Design review of the part built by this model. Coordinates are the model's own, in mm. Face numbers are marked on the shaded views. A direction names the side the tool comes from. Coordinates: 2 decimals unless noted, no trailing zeros. Order: outer loops, then holes, each group sorted by start corner. A loop starts at its lowest first (then second) coordinate and runs counter-clockwise, first axis right, second up. Notation, with made-up numbers: (-27.75, 7.25) -> (18.25, 7.25) arc R32 cw to (18.25, 34.25) -> close; hole circle Ø3 at (16.25, -3). An arc over 180 degrees is marked (long way). Write item = value, one per line.
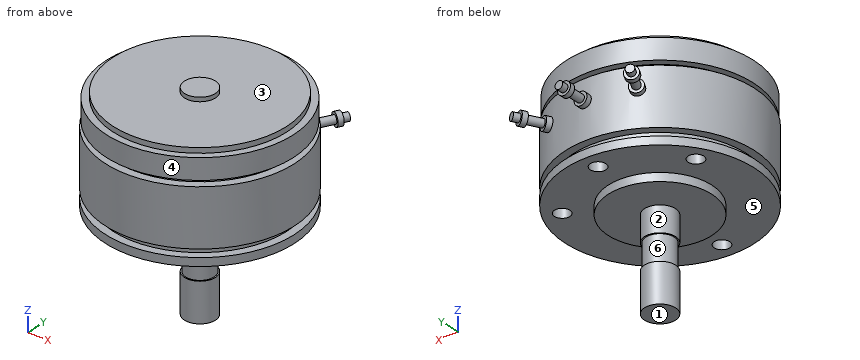
```python
from build123d import *

# Parameters (mm, degrees)
SKETCH_5_R                 = 3
SKETCH_5_R_2               = 2.75
EXTRUDE_3_DEPTH            = 19
SKETCH_5_3_R               = 10
SKETCH_5_3_R_2             = 3
EXTRUDE_4_DEPTH            = 1.6
CUT_EXTRUDE_START          = 6.5
SKETCH_5_4_R               = 3
SKETCH_5_4_R_2             = 2.75
CUT_EXTRUDE_5_DEPTH        = 5
SKETCH_6_R                 = 0.75
EXTRUDE_5_DEPTH            = 24.5
EXTRUDE_START              = 18.207141
SKETCH_6_4_R               = 1.25
SKETCH_6_4_R_2             = 0.75
EXTRUDE_10_DEPTH           = 5.042859
SKETCH_6_5_R               = 1.25
SKETCH_6_5_R_2             = 0.75
CUT_EXTRUDE_6_DEPTH        = 22.25
SKETCH_6_6_R               = 1.25
SKETCH_6_6_R_2             = 0.75
EXTRUDE_11_DEPTH           = 19.25
PATTERN_CIRCULAR_1_ANGLE   = 28
PATTERN_CIRCULAR_1_2_ANGLE = 28
SKETCH_7_R                 = 1.5
CUT_EXTRUDE_7_DEPTH        = 3
EXTRUDE_START_2            = 0.8
SKETCH_8_R                 = 3
EXTRUDE_12_DEPTH           = 0.8


with BuildPart() as part:
    # Sketch 4 → Revolve 1 (revolve)
    with BuildSketch(Plane(origin=(0, 0, 0), x_dir=(0, 0, -1), z_dir=(1, 0, 0)), mode=Mode.PRIVATE) as revolve_1_sk:
        Polygon((0, 0), (0, 16.75), (1, 16.75), (1, 18.05), (5, 18.05), (5, 16.75), (6, 16.75), (6, 18.25), (16.93, 18.25), (16.93, 16.75), (18.43, 16.75), (18.43, 18.25), (20, 18.25), (20, 0), align=None)
    revolve(revolve_1_sk.sketch.rotate(Axis((0, 0, 42.478286457), (0, 0, -1)), 90), axis=Axis((0, 0, 42.478286457), (0, 0, -1)))

    # Sketch 5 → Extrude 3 (add)
    # profile 1 of 2: a face of its own
    with BuildSketch(Plane(origin=(0, 0, -20), x_dir=(-1, 0, 0), z_dir=(0, 0, -1))):
        Circle(SKETCH_5_R)
        Circle(SKETCH_5_R_2, mode=Mode.SUBTRACT)
    # profile 2 of 2: a face of its own
    with BuildSketch(Plane(origin=(0, 0, -20), x_dir=(-1, 0, 0), z_dir=(0, 0, -1))):
        Circle(SKETCH_5_R_2)
    extrude(amount=EXTRUDE_3_DEPTH)

    # Sketch 5_3 → Extrude 4 (add)
    with BuildSketch(Plane(origin=(0, 0, -20), x_dir=(-1, 0, 0), z_dir=(0, 0, -1))):
        Circle(SKETCH_5_3_R)
        Circle(SKETCH_5_3_R_2, mode=Mode.SUBTRACT)
    extrude(amount=EXTRUDE_4_DEPTH)

    # Sketch 5_4 → Cut-Extrude 5 (cut)
    with BuildSketch(Plane(origin=(0, 0, -20), x_dir=(-1, 0, 0), z_dir=(0, 0, -1)).offset(CUT_EXTRUDE_START)):
        Circle(SKETCH_5_4_R)
        Circle(SKETCH_5_4_R_2, mode=Mode.SUBTRACT)
    extrude(amount=CUT_EXTRUDE_5_DEPTH, mode=Mode.SUBTRACT)

    # Sketch 6 → Extrude 5 (add)
    with BuildSketch(Plane(origin=(0, 0, 0), x_dir=(1, 0, 0), z_dir=(0, 1, 0))):
        with Locations(Location((0, 10, 0), (0, 0, 90))):
            Circle(SKETCH_6_R)
    extrude(amount=EXTRUDE_5_DEPTH)

    # Sketch 6_4 → Extrude 10 (add)
    with BuildSketch(Plane(origin=(0, 0, 0), x_dir=(1, 0, 0), z_dir=(0, 1, 0)).offset(EXTRUDE_START)):
        with Locations(Location((0, 10, 0), (0, 0, 90))):
            Circle(SKETCH_6_4_R)
        with Locations(Location((0, 10, 0), (0, 0, 270))):
            Circle(SKETCH_6_4_R_2, mode=Mode.SUBTRACT)
    extrude(amount=EXTRUDE_10_DEPTH)

    # Sketch 6_5 → Cut-Extrude 6 (cut)
    with BuildSketch(Plane(origin=(0, 0, 0), x_dir=(1, 0, 0), z_dir=(0, 1, 0))):
        with Locations(Location((0, 10, 0), (0, 0, 90))):
            Circle(SKETCH_6_5_R)
        with Locations(Location((0, 10, 0), (0, 0, 270))):
            Circle(SKETCH_6_5_R_2, mode=Mode.SUBTRACT)
    extrude(amount=CUT_EXTRUDE_6_DEPTH, mode=Mode.SUBTRACT)

    # Sketch 6_6 → Extrude 11 (add)
    with BuildSketch(Plane(origin=(0, 0, 0), x_dir=(1, 0, 0), z_dir=(0, 1, 0))):
        with Locations(Location((0, 10, 0), (0, 0, 90))):
            Circle(SKETCH_6_6_R)
        with Locations(Location((0, 10, 0), (0, 0, 270))):
            Circle(SKETCH_6_6_R_2, mode=Mode.SUBTRACT)
    extrude(amount=EXTRUDE_11_DEPTH)


with BuildPart() as body_2:
    # Pattern Circular 1: read off the stored shape, not the designer's step
    # Pattern Circular 1: copy of part
    add(part.part.rotate(Axis((0, 0, 0), (0, 0, -1)), PATTERN_CIRCULAR_1_ANGLE))


with BuildPart() as body_3:
    # Pattern Circular 1 2: copy of part
    add(part.part.rotate(Axis((0, 0, 0), (0, 0, 1)), PATTERN_CIRCULAR_1_2_ANGLE))


with BuildPart() as cut_extrude_7_tool:
    # Sketch 7 → Cut-Extrude 7 (new body)
    with BuildSketch(Plane(origin=(0, 0, -20), x_dir=(-1, 0, 0), z_dir=(0, 0, -1))):
        with Locations((0, 15)):
            Circle(SKETCH_7_R)
        with Locations(Location((0, -15, 0), (0, 0, 180))):
            Circle(SKETCH_7_R)
        with Locations(Location((-12.990381057, 7.5, 0), (0, 0, 180))):
            Circle(SKETCH_7_R)
        with Locations(Location((12.990381057, 7.5, 0), (0, 0, 180))):
            Circle(SKETCH_7_R)
    extrude(amount=-CUT_EXTRUDE_7_DEPTH)


with BuildPart() as part_1:
    add(part.part)

    # Cut-Extrude 7: cut by cut_extrude_7_tool
    add(cut_extrude_7_tool.part, mode=Mode.SUBTRACT)



with BuildPart() as body_2_1:
    add(body_2.part)

    # Cut-Extrude 7: cut by cut_extrude_7_tool
    add(cut_extrude_7_tool.part, mode=Mode.SUBTRACT)


with BuildPart() as body_3_1:
    add(body_3.part)

    # Cut-Extrude 7: cut by cut_extrude_7_tool
    add(cut_extrude_7_tool.part, mode=Mode.SUBTRACT)


with BuildPart() as part_2:
    add(part_1.part)

    add(body_2_1.part)  # Extrude 12 merges body 2

    add(body_3_1.part)  # Extrude 12 merges body 3
    # Sketch 8 → Extrude 12 (add)
    with BuildSketch(Plane.XY.offset(EXTRUDE_START_2)):
        with Locations(Location((0, 0, 0), (0, 0, 180))):
            Circle(SKETCH_8_R)
    extrude(amount=-EXTRUDE_12_DEPTH)


solid = part_2.part
```
(1) We need section A-A (x = 13). Write out the cut boundary in (y, z).
Report:
outline = (-12.81, -20) -> (6, -20) -> (6, -17) -> (9, -17) -> (9, -20) -> (12.81, -20) -> (12.81, -18.43) -> (10.56, -18.43) -> (10.56, -16.93) -> (12.81, -16.93) -> (12.81, -6) -> (10.56, -6) -> (10.56, -5) -> (12.52, -5) -> (12.52, -1) -> (10.56, -1) -> (10.56, 0) -> (-10.56, 0) -> (-10.56, -1) -> (-12.52, -1) -> (-12.52, -5) -> (-10.56, -5) -> (-10.56, -6) -> (-12.81, -6) -> (-12.81, -16.93) -> (-10.56, -16.93) -> (-10.56, -18.43) -> (-12.81, -18.43) -> close
(2) Insertion check: pin 1 (2.5 mm diameter, centred on x = 13, y = 7, fed in from -Z); pin 2 (8 mm diameter, centred on x = 8, z = -11.5, fed in from +Y); pin 3 (3 mm diameter, centred on x = 12, y = -2.5, fed in from +Z). Each pin has a flat end and moves straight along its axis. Give the tip position at first contact, or say it passes through.
Report:
pin_1 = -20
pin_2 = 21.98
pin_3 = 0
(3) For the marked faces 1 and 2, list the 3-axis set-ups (+Z, -Z, +X, -X, +Y, -Y) from which the entire face can be reached by the end or side of a thin tool; tool diameter is ignored.
Report:
face_1 = -Z, +X, -X, +Y, -Y
face_2 = -Z
(4) We need section C-C (z = -13.5). Write out the cut boundary in (x, y).
Report:
outline = circle Ø36.5 at (0, 0)
(5) The part is to be moulded in two halves that separate along Z. For the marked faces 3, 4, 5 and 6, say which applies: released by +Z, released by -Z, zero draft, split by the parting line, or undercut.
Report:
face_3 = released by +Z
face_4 = zero draft
face_5 = released by -Z
face_6 = undercut
(6) We need section D-D (z = -22.5). Write out the cut boundary in (x, y), and give its area (3 significant figures).
Report:
outline = circle Ø6 at (0, 0)
area = 28.3 mm²
(7) We need section B-B (y = -15). Write out the cut boundary in (x, z).
Report:
outline = (-10.4, -20) -> (-1.5, -20) -> (-1.5, -17) -> (1.5, -17) -> (1.5, -20) -> (10.4, -20) -> (10.4, -18.43) -> (7.45, -18.43) -> (7.45, -16.93) -> (10.4, -16.93) -> (10.4, -6) -> (7.45, -6) -> (7.45, -5) -> (10.04, -5) -> (10.04, -1) -> (7.45, -1) -> (7.45, 0) -> (-7.45, 0) -> (-7.45, -1) -> (-10.04, -1) -> (-10.04, -5) -> (-7.45, -5) -> (-7.45, -6) -> (-10.4, -6) -> (-10.4, -16.93) -> (-7.45, -16.93) -> (-7.45, -18.43) -> (-10.4, -18.43) -> close
(8) For L1, parallel to Y at x = 0, z = -18; L2, parallel to Y at x = 0, z = -19.4; L3, parallel to X at y = 7.5, z = -19, list the stretches that pass through material, from the lowest coordinate up.
Report:
L1 = -16.75 to -16.5, -13.5 to 13.5, 16.5 to 16.75
L2 = -18.25 to -16.5, -13.5 to 13.5, 16.5 to 18.25
L3 = -16.64 to -14.49, -11.49 to 11.49, 14.49 to 16.64
